Solid Edge part; units mm, degrees
sketch "Sketch1" plane through (0, 0, 0) normal (1, 0, 0) x (0, 1, 0)
  circle A0 centre (0, 0) radius 4
extrude "Protrusion1" add sketch "Sketch1" against normal blind 250
sketch "Sketch2" plane through (0, 0, 0) normal (1, 0, 0) x (0, 1, 0)
  line L0 (-6.0933, 1.2954) -> (6.7659, 1.2954)
  line L1 (6.7659, 1.2954) -> (6.7659, -1.2046)
  line L2 (6.7659, -1.2046) -> (-6.2341, -1.2046)
  line L3 (-6.2341, -1.2046) -> (-6.2341, 1.2954)
  line L4 (-6.2341, 1.2954) -> (-6.0933, 1.2954)
  dimension "D1" = 6.7659
extrude "拉伸_6" add sketch "Sketch2" against normal blind 15
sketch "Sketch3" plane through (-7.5, -6.2341, 0.0454) normal (0, -1, 0) x (1, 0, 0)
  line L0 (7.5, 1.25) -> (2.5, 1.25)
  line L1 (2.5, 1.25) -> (2.5, -1.25)
  line L2 (2.5, -1.25) -> (7.5, -1.25)
  line L3 (7.5, -1.25) -> (7.5, 1.25)
extrude "拉伸除料_1" cut sketch "Sketch3" against normal blind 2.5
sketch "Sketch4" plane through (-7.5, 5.2752, 1.2954) normal (0, 0, 1) x (1, 0, 0)
  line L0 (7.5, 1.4908) -> (2.5, 1.4908)
  line L1 (2.5, 1.4908) -> (2.5, -1.4908)
  line L2 (2.5, -1.4908) -> (7.5, -1.4908)
  line L3 (7.5, -1.4908) -> (7.5, 1.4908)
extrude "Cutout1" cut sketch "Sketch4" against normal blind 2.5
sketch "Sketch5" plane through (0, 0, 0) normal (0, -1, 0) x (1, 0, 0)
  line L0 (-250, 4) -> (-235, 4)
  line L1 (-235, 4) -> (-250, 1)
  line L2 (-250, 1) -> (-250, 4)
  dimension "D1" = 250
  dimension "D2" = 235
extrude "Cutout2" cut sketch "Sketch5" against normal blind 21.4935
sketch "Sketch6" plane through (0, 0, 0) normal (0, -1, 0) x (1, 0, 0)
  line L0 (-250, 4) -> (-235, 4)
  line L1 (-235, 4) -> (-250, 1)
  line L2 (-250, 1) -> (-250, 4)
  dimension "D1" = 250
extrude "拉伸除料_4" cut sketch "Sketch6" along normal blind 51.5804
sketch "Sketch7" plane through (0, 0, 0) normal (0, -1, 0) x (1, 0, 0)
  line L0 (-250, -4) -> (-250, -1)
  line L1 (-250, -1) -> (-235, -4)
  line L2 (-235, -4) -> (-250, -4)
  dimension "D1" = 250
  dimension "D2" = 235
extrude "拉伸除料_5" cut sketch "Sketch7" along normal blind 13.6842
sketch "Sketch8" plane through (-242.5, 0, -2.5) normal (0, -1, 0) x (1, 0, 0)
  line L0 (-7.5, 1.5) -> (-7.5, -1.5)
  line L1 (-7.5, -1.5) -> (7.5, -1.5)
  line L2 (7.5, -1.5) -> (-7.5, 1.5)
extrude "Cutout3" cut sketch "Sketch8" against normal blind 26.2163
properties material "不锈钢 303"
Here's how the part is built. I have some questions about the finished solid (model axes, mm). A direction names the side the tool comes from. Give positions to 0.01 mm unless a question says otherwise; leave off trailing zeros. Order: outer loops, then holes, each group sorted by start corner. A loop starts at its lowest first (then second) coordinate and runs counter-clockwise, first axis right, second up. Notation, with made-up numbers: (-7.5, -9) -> (47.5, -9) arc R30 cw to (47.5, 18) -> close; hole circle Ø5 at (45.25, 76). An arc over 180 degrees is marked (long way). Use a Markdown table: item, result. Add a question column.
Item 1: For faces 1 (the face through (-123.25, -0.867, -3.905)), 2 (the face through (-244.06, 0.05, 2.19)), which set-ups out of +Z, -Z, +X, -X, +Y, -Y let a thin tool reach every point of the face, with its end or its side?
Item 2: Imagine slicing it at C-C on z = 2.5. Please give me the cut outline in (x, y), plus the area to 3 significant figures.
Item 3: I need wall thicknesses on line 1 (Y direction, x = -216, z = 0.5); line 2 (Y direction, x = -239, z = 1). Which ranges of each line are inside material? Lowest first, please.
Item 4: Will these pins go through, and if not, where does the flat tip stop? pin 1 (2 mm diameter, centred on y = 6, z = 0, fed in from +X); pin 2 (0.8 mm diameter, centred on y = 5.5, z = 0.5, fed in from -X); pin 3 (1.9 mm diameter, centred on x = -12, y = -5, fed in from -Z); pin 4 (2.5 mm diameter, centred on y = -4.5, z = 0.5, fed in from +X).
Item 5: Imagine slicing it at A-A on y = 0. Please give me the cut outline in (x, z).
Item 6: Imagine slicing it at B-B on x = -119. Please give me the cut outline in (y, z), plus the area to 3 significant figures.
Data:
| question | item | result |
|---|---|---|
| 1 | face 1 | -X |
| 1 | face 2 | +Z, -X, +Y, -Y |
| 2 | outline | (-242.5, -3.12) -> (0, -3.12) -> (0, 3.12) -> (-242.5, 3.12) -> close |
| 2 | area | 1,510 mm² |
| 3 | line 1 | y = -3.97 to 3.97 |
| 3 | line 2 | y = -3.87 to 3.87 |
| 4 | pin 1 | stops at x = -5 |
| 4 | pin 2 | stops at x = -15 |
| 4 | pin 3 | stops at z = -1.2 |
| 4 | pin 4 | stops at x = 0 |
| 5 | outline | (-250, -1) -> (-235, -4) -> (0, -4) -> (0, 4) -> (-235, 4) -> (-250, 1) -> close |
| 6 | outline | circle Ø8 at (0, 0) |
| 6 | area | 50.3 mm² |
